```python
from build123d import *

# Parameters (mm, degrees)
F1_DEPTH = 18
F0_W     = 520
F0_H     = 85
F2_DEPTH = 15


with BuildPart() as f1:
    # F0 (on Front) → F1 (new body)
    with BuildSketch(Plane.XZ):
        Polygon((-260, -150), (260, -150), (211.875, 235), (-260, 235), align=None)
    extrude(amount=-F1_DEPTH)



with BuildPart() as f1b:
    # F0 (on Front) → F1, piece 2 (new body)
    with BuildSketch(Plane.XZ):
        with Locations((0, -207.5)):
            Rectangle(F0_W, F0_H)
    extrude(amount=-F1_DEPTH)


with BuildPart() as f1_1:
    add(f1.part)

    add(f1b.part)  # F2 merges F1b
    # F0 (on Front) → F2 (join)
    with BuildSketch(Plane.XZ):
        Polygon((275, -150), (225, 250), (-275, 250), (-275, -250), (-260, -250), (-260, -165), (260, -165), (260, -250), (275, -250), align=None)
        Polygon((211.875, 235), (260, -150), (-260, -150), (-260, 235), align=None, mode=Mode.SUBTRACT)
    extrude(amount=-F2_DEPTH)


solid = f1_1.part
```
The model under review builds one solid part; all positions refer to its coordinate system, in mm. A direction names the side the tool comes from. Give positions to 0.01 mm unless a question says otherwise; leave off trailing zeros. Write each loop counter-clockwise with the first axis right and the second up, starting at its lowest first coordinate (ties: lowest second). Pieces come first, ordered by that corner, then holes. Notation, with made-up numbers: M 2,-25 L 22,-25 A28 ccw 22,-6 Z; hole C -38,35 d9. An arc over 180 degrees is marked long. Answer in a Markdown table with one row per item.
Item 1: Add section C-C on z = 68. Give the boundary of the cut face in (x, y).
Check sheet entries:
| item | result |
|---|---|
| outline | M -275,0 L 247.75,0 L 247.75,15 L 232.75,15 L 232.75,18 L -260,18 L -260,15 L -275,15 Z |
Item 2: Tool access review of faces 1 (the face through (236.274, 16.479, 39.805)), 2 (the face through (-4, 9, -250)): name each direction out of +Z, -Z, +X, -X, +Y, -Y from which nothing blocks a thin tool from reaching the whole face with its end or side.
Check sheet entries:
| item | result |
|---|---|
| face 1 | +Z, +X, +Y |
| face 2 | -Z, +X, -X, +Y, -Y |
Item 3: Add section A-A on z = -120. Give the boundary of the cut face in (x, y), plus the area to 3 significant figures.
Check sheet entries:
| item | result |
|---|---|
| outline | M -275,0 L 271.25,0 L 271.25,15 L 256.25,15 L 256.25,18 L -260,18 L -260,15 L -275,15 Z |
| area | 9,740 mm2 |
Item 4: For P1, Ø1.5, axis at y = 16, z = -2, coming from the -X side; P2, Ø2, axis at y = 13.5, z = 198, coming from the +X side (3 decimals); P3, Ø2.5, axis at x = -68.5, y = 16.5, coming from the +Z side, all flat-tipped, find the tip position at first contact; note any pin that passes through.
Check sheet entries:
| item | result |
|---|---|
| P1 | x = -260 |
| P2 | x = 231.625 |
| P3 | z = 235 |
Item 5: Add section B-B on y = 9.5. Give the boundary of the cut face in (x, z), plus the area to 3 significant figures.
Check sheet entries:
| item | result |
|---|---|
| outline | M -275,-250 L 275,-250 L 275,-150 L 225,250 L -275,250 Z |
| area | 265,000 mm2 |
Item 6: For line 1 along X through (y, z) = (9, -10.5); line 2 along X through (y, z) = (3.75, 168); line 3 along Y through (x, z) = (-77.5, -153), list the stretches that pass through material, from the lowest coordinate up.
Check sheet entries:
| item | result |
|---|---|
| line 1 | -275 to 257.56 |
| line 2 | -275 to 235.25 |
| line 3 | 0 to 15 |
